Geometry: final body of the model. Coordinates: model frame, mm. A direction names the side the tool comes from. Coordinates: 2 decimals unless noted, no trailing zeros. Loops run counter-clockwise (first coordinate to the right, second up) from the corner with the lowest first, then second, coordinate; pieces in that order, holes last. Notation, with made-up numbers: M -23.75,80 L -8.75,80 A25 ccw -8.75,106 Z; hole C 76.25,29 d6. An arc over 180 degrees is marked long. Write each question's results on one line, items separated by ' | '. Start each with the question number.
from build123d import *

# Parameters (mm, degrees)
SKETCH1_W                   = 69.85
SKETCH1_H                   = 101.6
BASE_FLANGE1_DEPTH          = 3.175
EDGE_FLANGE1_DEPTH          = 69.85
F_5_0_2055_DIAMETER_HOLE1_D = 5.2197
F_5_0_2055_DIAMETER_HOLE3_D = 5.2197
SKETCH21_R                  = 2.60985
CUT_EXTRUDE1_DEPTH          = 126.88384527


# Sheet-metal steps are written as plain solids
with BuildPart() as part:
    # Sketch1 → Base-Flange1 (new body)
    with BuildSketch(Plane(origin=(0, 0, 0), x_dir=(1, 0, 0), z_dir=(0, 1, 0))):
        with Locations((34.925, 50.8)):
            Rectangle(SKETCH1_W, SKETCH1_H)
    extrude(amount=-BASE_FLANGE1_DEPTH)

    # Edge-Flange1 section (across the edge) → Edge-Flange1 (add)
    with BuildSketch(Plane(origin=(0, 0, 3.9116), x_dir=(0, 0, -1), z_dir=(1, 0, 0))):
        with BuildLine():
            Line((-3.175, 0.7366), (-3.175, 22.225))
            Line((-3.175, 22.225), (0, 22.225))
            Line((0, 22.225), (0, 0.7366))
            ThreePointArc((0, 0.7366), (0.215745145, 0.215745145), (0.7366, 0))
            Line((0.7366, 0), (3.9116, 0))
            Line((3.9116, 0), (3.9116, -3.175))
            Line((3.9116, -3.175), (0.7366, -3.175))
            ThreePointArc((0.7366, -3.175), (-2.029318885, -2.029318885), (-3.175, 0.7366))
        make_face()
    extrude(amount=EDGE_FLANGE1_DEPTH)

    # #5 (0.2055) Diameter Hole1 (through all)
    with Locations(Plane.XZ.offset(3.175)):
        with Locations((33.3375, -34.1884), (23.8125, -62.7634), (33.3375, -72.2884), (57.15, -84.9884), (57.15, -40.5384), (9.525, -40.5384), (9.525, -84.9884)):
            Hole(F_5_0_2055_DIAMETER_HOLE1_D / 2)

    # #5 (0.2055) Diameter Hole3 (through all)
    with Locations(Plane.XY.offset(7.0866)):
        with Locations((6.35, 12.7), (19.05, 12.7), (31.75, 12.7), (44.45, 12.7), (57.15, 12.7)):
            Hole(F_5_0_2055_DIAMETER_HOLE3_D / 2)

    # Sketch21 → Cut-Extrude1 (cut, through all)
    with BuildSketch(Plane.XZ.offset(3.175)):
        with Locations(Location((19.050000049, -11.9634, 0), (0, 0, 270))):
            Circle(SKETCH21_R)
        with Locations(Location((6.350000049, -11.9634, 0), (0, 0, 270))):
            Circle(SKETCH21_R)
        with Locations(Location((31.750000049, -11.9634, 0), (0, 0, 270))):
            Circle(SKETCH21_R)
        with Locations(Location((44.450000049, -11.9634, 0), (0, 0, 270))):
            Circle(SKETCH21_R)
        with Locations(Location((57.150000049, -11.9634, 0), (0, 0, 270))):
            Circle(SKETCH21_R)
    extrude(amount=-CUT_EXTRUDE1_DEPTH, mode=Mode.SUBTRACT)


solid = part.part
Item 1: Ray query, L1, parallel to Z at x = 47.5, y = 15.25; L2, parallel to Y at x = 3.5, z = -42.5 (3 decimals); L3, parallel to Z at x = 59.5, y = 0.25. Return the intervals inside material, ascending. Write a range as [from, to].
Item 2: Set-up query: faces 4 (the flat face through (34, 0, -48)), 5 (the flat face through (34, 11, 7.087)). Return all of +Z, -Z, +X, -X, +Y, -Y with unobstructed straight access to the full face (end or side cutting, diameter ignored); none if empty.
Item 3: Contact query for flat-ended pins moving along their axis: P1, Ø7, axis at x = 19.05, z = -11.96, coming from the +Y side; P2, Ø6.5, axis at x = 44.5, y = 15.5, coming from the -Z side. Output: stop coordinate, or through.
Item 4: Pull-direction query (X, two-part tool) for faces 1 (the flat face through (0, -1, -35)), 2 (the cylindrical face through (59.757, 12.815, 5.477)), 3 (the flat face through (34, -3.175, -50)); classes: released by +X, released by -X, zero draft, split by the parting line, or undercut.
Item 5: Section A-A, the plane y = 12.7. Return loops of the section in (x, z), plus the area to 3 significant figures.
Item 6: Section B-B, the plane x = 57.15. Return loops of the section in (y, z) (3 decimals), plus the area to 3 significant figures.
Item 7: Section D-D, the plane z = -35.5. Return loops of the section in (x, y) (3 decimals), plus the area to 3 significant figures.
Item 8: Section C-C, the plane x = 19.05. Return loops of the section in (y, z) (3 decimals), plus the area to 3 significant figures.
Solutions:
1) L1: z = [3.91, 7.09] | L2: y = [-3.175, 0] | L3: z = [3.73, 7.06]
2) face 4: -Z, +X, -X, +Y | face 5: +Z, +X, -X, +Y, -Y
3) P1: stops at y = 0 | P2: stops at z = 3.91
4) face 1: released by -X | face 2: undercut | face 3: zero draft
5) outline: M 0,3.91 L 3.74,3.91 L 3.74,7.09 L 0,7.09 Z; M 8.96,3.91 L 16.44,3.91 L 16.44,7.09 L 8.96,7.09 Z; M 21.66,3.91 L 29.14,3.91 L 29.14,7.09 L 21.66,7.09 Z; M 34.36,3.91 L 41.84,3.91 L 41.84,7.09 L 34.36,7.09 Z; M 47.06,3.91 L 54.54,3.91 L 54.54,7.09 L 47.06,7.09 Z; M 59.76,3.91 L 69.85,3.91 L 69.85,7.09 L 59.76,7.09 Z | area: 139 mm²
6) outline: M -3.175,-101.6 L 0,-101.6 L 0,-87.598 L -3.175,-87.598 Z; M -3.175,-82.379 L 0,-82.379 L 0,-43.148 L -3.175,-43.148 Z; M -3.175,-37.929 L 0,-37.929 L 0,-14.573 L -3.175,-14.573 Z; M -3.175,-9.354 L 0,-9.354 L 0,3.175 A0.737 cw 0.737,3.912 L 10.09,3.912 L 10.09,7.087 L 0.737,7.087 A3.912 ccw -3.175,3.175 Z; M 15.31,3.912 L 22.225,3.912 L 22.225,7.087 L 15.31,7.087 Z | area: 346 mm²
7) outline: M 0,-3.175 L 31.081,-3.175 L 31.081,0 L 0,0 Z; M 35.594,-3.175 L 69.85,-3.175 L 69.85,0 L 35.594,0 Z | area: 207 mm²
8) outline: M -3.175,-101.6 L 0,-101.6 L 0,-14.573 L -3.175,-14.573 Z; M -3.175,-9.354 L 0,-9.354 L 0,3.175 A0.737 cw 0.737,3.912 L 10.09,3.912 L 10.09,7.087 L 0.737,7.087 A3.912 ccw -3.175,3.175 Z; M 15.31,3.912 L 22.225,3.912 L 22.225,7.087 L 15.31,7.087 Z | area: 379 mm²
